Read the model definition and answer for the solid it produces. Units are mm, in the model's axes. Coordinates: 2 decimals unless noted, no trailing zeros. Loops run counter-clockwise (first coordinate to the right, second up) from the corner with the lowest first, then second, coordinate; pieces in that order, holes last. Notation, with made-up numbers: M 12,-15.5 L 65,-15.5 A29 cw 65,13.5 Z; hole C -21,58 d8. An arc over 180 degrees is marked long. Use one line per item in the form item = value. Start each with the question number.
1. The part is cut by section D-D (x = -2.54). Give the vertices of the cut face in (y, z), plus the area to 3 significant figures.
2. The part is cut by section B-B (z = -0.6). Give the vertices of the cut face in (x, y) (3 decimals), plus the area to 3 significant figures.
3. For a pull along X with two mould halves and no side action, classify faces 1 (the flat face through (0, 2, 2)), 2 (the flat face through (0, 3.7, 0)), 3 (the flat face through (-4.315, 2, 0)) as released by +X, released by -X, zero draft, split by the parting line, or undercut.
4. The part is cut by section C-C (y = 5.5). Give the vertices of the cut face in (x, z).
5. Flat-ended cylindrical pins translate along their axes: pin 1 (1.5 mm diameter, centred on x = -0.5, z = 0, fed in from +Y); pin 2 (2 mm diameter, centred on x = -1.5, z = -0.5, fed in from +Y); pin 3 (0.5 mm diameter, centred on y = 5, z = 0, fed in from +X); pin 4 (0.8 mm diameter, centred on x = 1, y = 5.5, fed in from -Z). Find the tip coordinate at first contact, or state that the pin passes through.
6. The part is cut by section A-A (x = 0). Give the vertices of the cut face in (y, z), plus the area to 3 significant figures.
7. Find the intervals of material crossed by probe 1 along Y at (x, z) = (0.75, 1.45); probe 2 along X at (y, z) = (4, 0); probe 3 along Y at (x, z) = (1.75, -0.65), in increasing order. Write a range as [from, to].
from build123d import *

# Parameters (mm, degrees)
SKETCH_1_W          = 8.63
SKETCH_1_H          = 4
EXTRUDE_1_DEPTH     = 3.8
SKETCH_2_W          = 3.8
SKETCH_2_H          = 1.9
CUT_EXTRUDE_1_DEPTH = 0.1
SKETCH_3_W          = 1.6
SKETCH_3_H          = 1.6
EXTRUDE_2_DEPTH     = 2.8
SKETCH_4_R          = 0.2
EXTRUDE_3_DEPTH     = 2


with BuildPart() as part:
    # Эскиз1 → Бобышка-Вытянуть1 (new body)
    with BuildSketch(Plane(origin=(0, 0, 0), x_dir=(1, 0, 0), z_dir=(0, 1, 0))):
        Rectangle(SKETCH_1_W, SKETCH_1_H)
    extrude(amount=EXTRUDE_1_DEPTH)

    # Эскиз2 → Вырез-Вытянуть1 (cut)
    with BuildSketch(Plane(origin=(0, 3.8, 0), x_dir=(1, 0, 0), z_dir=(0, 1, 0))):
        Rectangle(SKETCH_2_W, SKETCH_2_H)
    extrude(amount=-CUT_EXTRUDE_1_DEPTH, mode=Mode.SUBTRACT)

    # Эскиз3 → Бобышка-Вытянуть2 (add)
    with BuildSketch(Plane(origin=(0, 3.7, 0), x_dir=(1, 0, 0), z_dir=(0, 1, 0))):
        with Locations((1.01593525, 0)):
            Rectangle(SKETCH_3_W, SKETCH_3_H)
    extrude(amount=EXTRUDE_2_DEPTH)

    # Эскиз4 → Бобышка-Вытянуть3 (add)
    with BuildSketch(Plane.XZ):
        with Locations((-2.54, 0)):
            Circle(SKETCH_4_R)
        Circle(SKETCH_4_R)
        with Locations((2.54, 0)):
            Circle(SKETCH_4_R)
    extrude(amount=EXTRUDE_3_DEPTH)


solid = part.part
Computed values:
q1.outline = M -2,-0.2 L 0,-0.2 L 0,-2 L 3.8,-2 L 3.8,2 L 0,2 L 0,0.2 L -2,0.2 Z
q1.area = 16.0 mm²
q2.outline = M -4.315,0 L 4.315,0 L 4.315,3.8 L 1.9,3.8 L 1.9,3.7 L 1.816,3.7 L 1.816,6.5 L 0.216,6.5 L 0.216,3.7 L -1.9,3.7 L -1.9,3.8 L -4.315,3.8 Z
q2.area = 36.9 mm²
q3.face_1 = zero draft
q3.face_2 = undercut
q3.face_3 = released by -X
q4.outline = M 0.22,-0.8 L 1.82,-0.8 L 1.82,0.8 L 0.22,0.8 Z
q5.pin_1 = 6.5
q5.pin_2 = 3.8
q5.pin_3 = 1.82
q5.pin_4 = -0.8
q6.outline = M -2,-0.2 L 0,-0.2 L 0,-2 L 3.8,-2 L 3.8,-0.95 L 3.7,-0.95 L 3.7,0.95 L 3.8,0.95 L 3.8,2 L 0,2 L 0,0.2 L -2,0.2 Z
q6.area = 15.8 mm²
q7.probe_1 = [0, 3.8]
q7.probe_2 = [0.22, 1.82]
q7.probe_3 = [0, 6.5]
